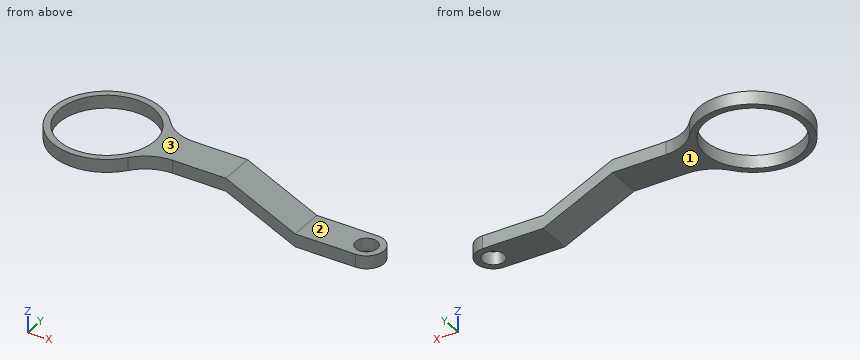
Autodesk Inventor part; units mm, degrees
ref_plane "Work Plane3" through (0, 0, 0) normal (0, 1, 0) x (-1, 0, 0)
ref_plane "YZ Plane" through (0, 0, 0) normal (1, 0, 0) x (0, 1, 0)
ref_plane "XY Plane" through (0, 0, 0) normal (0, 0, 1) x (1, 0, 0)
sketch "Sketch1" plane through (0, 0, 0) normal (0, 0, 1) x (1, 0, 0)
  arc A0 (9.7855, 7.7778) -> (9.7855, -7.7778) centre (0, 0) ccw
  circle A1 centre (0, 0) radius 11
  arc A2 (60, -4) -> (60, 4) centre (60, 0) ccw
  line L0 (60, 4) -> (17.6139, 4) construction
  line L1 (60, -4) -> (17.6139, -4) construction
  arc A3 (17.6139, -4) -> (9.7855, -7.7778) centre (17.6139, -14) ccw
  arc A4 (9.7855, 7.7778) -> (17.6139, 4) centre (17.6139, 14) ccw
  line L2 (30, 4) -> (30, -4) construction
  line L3 (17.6139, -4) -> (17.6139, 4)
  point P0 (11.8427, 4)
  point P1 (11.8427, -4)
  point P2 (-12.5, 0)
  point P3 (30, 0)
  dimension "d0" = 25
  dimension "d1" = 22
  dimension "d2" = 4
  dimension "d3" = 10
  dimension "d4" = 60
  dimension "d17" = 42.5
extrude "Extrusion1" add sketch "Sketch1" against normal blind 3
ref_plane "Work Plane3" through (0, 0, 0) normal (0, 1, 0) x (-1, 0, 0)
sketch "Sketch7" plane through (0, 0, 0) normal (0, 1, 0) x (-1, 0, 0)
  line L0 (-17.6139, 0) -> (-17.6139, -3)
  line L1 (-17.6139, -3) -> (-30, -3)
  line L2 (-30, -3) -> (-46, -10.5)
  line L3 (-46, -10.5) -> (-60, -10.5)
  line L4 (-60, -10.5) -> (-60, -7.5)
  line L5 (-60, -7.5) -> (-46, -7.5)
  line L6 (-46, -7.5) -> (-30, 0)
  line L7 (-30, 0) -> (-17.6139, 0)
  line L8 (-17.6139, -3) -> (-17.6139, 0)
  point P0 (0, 0)
  point P1 (-60, -9)
  dimension "d19" = 7.5
  dimension "d20" = 14
  dimension "d21" = 60
  dimension "d22" = 3
extrude "Extrusion3" add sketch "Sketch7" along normal mid plane 8
sketch "Sketch8" plane through (46, 4, -7.5) normal (0, 0, 1) x (1, 0, 0)
  line L0 (14, -8) -> (14, 0)
  arc A0 (14, -8) -> (14, 0) centre (14, -4) ccw
  point P0 (-46, -4)
  dimension "d25" = 4
extrude "Extrusion4" add sketch "Sketch8" against normal up to surface (3 mm away)
sketch "Sketch9" plane through (46, -4, -7.5) normal (0, 0, 1) x (1, 0, 0)
  arc A0 (14, 0) -> (14, 8) centre (14, 4) ccw
  point P0 (-46, 4)
hole "Hole1" at (60, 0, -7.5) direction (0, 0, -1) diameter 5 depth 3
properties part number "15_3"
Geometry: final body of the model. Coordinates: model frame, mm. Face numbers are marked on the shaded views. A direction names the side the tool comes from. Give positions to 0.01 mm unless a question says otherwise; leave off trailing zeros. Order: outer loops, then holes, each group sorted by start corner. A loop starts at its lowest first (then second) coordinate and runs counter-clockwise, first axis right, second up. Notation, with made-up numbers: (69, 37) - (81, 37) arc R12 ccw to (81, 56) - close; hole circle Ø5 at (31, 4.5). An arc over 180 degrees is marked (long way). Use CSV: the item, a comma, the result in double quotes.
1. Material intervals for line 1 along Y through (x, z) = (0, -2); line 2 along Y through (x, z) = (60, -8.85); line 3 along Z through (x, y) = (7, 9.25), sorted ascending. Write a range as from..to.
Answers below:
line 1,"-12.5..-11, 11..12.5"
line 2,"-4..-2.5, 2.5..4"
line 3,"-3..0"
2. Section query A-A (x = 0). Output: boundary loops of the cut face in (y, z), plus the area to 3 significant figures.
Answers below:
outline,"(-12.5, -3) - (-11, -3) - (-11, 0) - (-12.5, 0) - close; (11, -3) - (12.5, -3) - (12.5, 0) - (11, 0) - close"
area,"9.00 mm2"
3. Section query D-D (z = -8.5). Output: boundary loops of the cut face in (x, y), plus the area to 3 significant figures.
Answers below:
outline,"(41.73, -4) - (60, -4) arc R4 ccw to (60, 4) - (41.73, 4) - close; hole circle Ø5 at (60, 0)"
area,"152 mm2"
4. Section query B-B (y = -5.5). Output: boundary loops of the cut face in (x, z).
Answers below:
outline,"(-11.22, -3) - (-9.53, -3) - (-9.53, 0) - (-11.22, 0) - close; (9.53, -3) - (12.35, -3) - (12.35, 0) - (9.53, 0) - close"
5. Section query C-C (y = 0). Output: boundary loops of the cut face in (x, z), plus the area to 4 significant figures.
Answers below:
outline,"(-12.5, -3) - (-11, -3) - (-11, 0) - (-12.5, 0) - close; (11, -3) - (30, -3) - (46, -10.5) - (57.5, -10.5) - (57.5, -7.5) - (46, -7.5) - (30, 0) - (11, 0) - close; (62.5, -10.5) - (64, -10.5) - (64, -7.5) - (62.5, -7.5) - close"
area,"148.5 mm2"
6. Access query for the marked faces 1, 2 and 3. Directions: +Z, -Z, +X, -X, +Y, -Y. A direction counts if a zero-diameter tool reaches every point of the face in a straight line with its end or side. Return the directions, or none.
Answers below:
face 1,"-Z, -X, +Y, -Y"
face 2,"+Z, +X, +Y, -Y"
face 3,"+Z, +X, -X, +Y, -Y"
7. Contact query for flat-ended pins moving along their axis: pin 1 (5 mm diameter, centred on x = 44, z = -3, fed in from -Y); pin 2 (1.5 mm diameter, centred on x = 26, y = 2.5, fed in from +Z); pin 3 (6.5 mm diameter, centred on x = 59, y = -1.5, fed in from +Z); pin 4 (12 mm diameter, centred on x = 23.5, y = -2, fed in from -Z). Output: stop coordinate, or through.
Answers below:
pin 1,"through"
pin 2,"z = 0"
pin 3,"z = -7.5"
pin 4,"z = -3"
